from build123d import *
from build123d.topology import SkipClean

# Parameters (mm, degrees)
SKETCH2_W           = 31.75
SKETCH2_H           = 6.35
BOSS_EXTRUDE2_DEPTH = 31.75
SKETCH3_W           = 19.999999878
SKETCH3_H           = 40.64
CUT_EXTRUDE1_DEPTH  = 37.061067996
SKETCH4_R           = 1.63195
CUT_EXTRUDE2_DEPTH  = 37.061067996
SKETCH7_W           = 3.175
SKETCH7_H           = 1.905
SKETCH7_W_2         = 2.54
SKETCH7_H_2         = 3.175
CUT_EXTRUDE4_DEPTH  = 37.061067996
CHAMFER1_SIZE       = 1.27
CUT_EXTRUDE3_DEPTH  = 2.38125
BOSS_EXTRUDE5_DEPTH = 31.75
SKETCH12_W          = 19.999999878
SKETCH12_H          = 25.4
CUT_EXTRUDE5_DEPTH  = 81.946934778
BOSS_EXTRUDE6_DEPTH = 9.071430469
BOSS_EXTRUDE7_DEPTH = 9.071428449
BOSS_EXTRUDE8_DEPTH = 31.75
SKETCH16_W          = 19.999999878
SKETCH16_H          = 45.357142858
SKETCH18_W          = 19.999999878
SKETCH18_H          = 38.1


with BuildPart() as part:
    # Sketch2 → Boss-Extrude2 (new, symmetric)
    with BuildSketch(Plane.XY):
        Rectangle(SKETCH2_W, SKETCH2_H)
    extrude(amount=BOSS_EXTRUDE2_DEPTH, both=True)

    # Sketch3 → Cut-Extrude1 (cut, through all)
    with BuildSketch(Plane(origin=(0, 3.175, 0), x_dir=(1, 0, 0), z_dir=(0, 1, 0))):
        Rectangle(SKETCH3_W, SKETCH3_H)
    extrude(amount=-CUT_EXTRUDE1_DEPTH, mode=Mode.SUBTRACT)

    # Sketch4 → Cut-Extrude2 (cut, through all)
    with BuildSketch(Plane(origin=(0, 3.175, 0), x_dir=(1, 0, 0), z_dir=(0, 1, 0))):
        with Locations(Location((-5.08, 25.4, 0), (0, 0, 270))):
            Circle(SKETCH4_R)
        with Locations(Location((5.08, 25.4, 0), (0, 0, 270))):
            Circle(SKETCH4_R)
        with Locations(Location((-5.08, -25.4, 0), (0, 0, 270))):
            Circle(SKETCH4_R)
        with Locations(Location((5.08, -25.4, 0), (0, 0, 270))):
            Circle(SKETCH4_R)
    extrude(amount=-CUT_EXTRUDE2_DEPTH, mode=Mode.SUBTRACT)

    # Sketch7 → Cut-Extrude4 (cut, through all)
    with BuildSketch(Plane(origin=(0, 3.175, 0), x_dir=(1, 0, 0), z_dir=(0, 1, 0))):
        with Locations((-2.8575, 21.2725)):
            Rectangle(SKETCH7_W, SKETCH7_H)
        with Locations((2.8575, 21.2725)):
            Rectangle(SKETCH7_W, SKETCH7_H)
        with Locations((2.8575, -21.2725)):
            Rectangle(SKETCH7_W, SKETCH7_H)
        with Locations((-2.8575, -21.2725)):
            Rectangle(SKETCH7_W, SKETCH7_H)
        with Locations((0, 21.2725)):
            Rectangle(SKETCH7_W_2, SKETCH7_H)
        with Locations((0, 23.8125)):
            Rectangle(SKETCH7_W_2, SKETCH7_H_2)
        with Locations((0, -21.2725)):
            Rectangle(SKETCH7_W_2, SKETCH7_H)
        with Locations((0, -23.8125)):
            Rectangle(SKETCH7_W_2, SKETCH7_H_2)
    extrude(amount=-CUT_EXTRUDE4_DEPTH, mode=Mode.SUBTRACT)

    # Chamfer1
    chamfer1_edges = [part.edges().sort_by_distance(p)[0] for p in [
        (-4.445, 0, -22.225),
        (4.445, 0, -22.225),
        (4.445, 0, 22.225),
        (-4.445, 0, 22.225),
    ]]
    chamfer(chamfer1_edges, length=CHAMFER1_SIZE)

    # Sketch6 → Cut-Extrude3 (cut)
    with BuildSketch(Plane.XZ.offset(3.175)):
        Polygon((-1.905, 27.233087105), (-5.08, 29.066174209), (-8.255, 27.233087105), (-8.255, 23.566912895), (-5.08, 21.733825791), (-1.905, 23.566912895), align=None)
        Polygon((8.255, 27.233087105), (5.08, 29.066174209), (1.905, 27.233087105), (1.905, 23.566912895), (5.08, 21.733825791), (8.255, 23.566912895), align=None)
        Polygon((8.255, -23.566912895), (5.08, -21.733825791), (1.905, -23.566912895), (1.905, -27.233087105), (5.08, -29.066174209), (8.255, -27.233087105), align=None)
        Polygon((-1.905, -23.566912895), (-5.08, -21.733825791), (-8.255, -23.566912895), (-8.255, -27.233087105), (-5.08, -29.066174209), (-1.905, -27.233087105), align=None)
    extrude(amount=-CUT_EXTRUDE3_DEPTH, mode=Mode.SUBTRACT)

    # Sketch10 → Boss-Extrude5 (add, through all)
    with BuildSketch(Plane(origin=(15.875, 0, 0), x_dir=(0, 0, -1), z_dir=(1, 0, 0))):
        Polygon((25.4, -47.625), (19.05, -47.625), (19.05, -34.925), (-19.05, -34.925), (-19.05, -47.625), (-25.4, -47.625), (-31.75, -3.175), (-22.678571429, -3.175), (-19.05, -28.575), (19.05, -28.575), (22.678571429, -3.175), (31.75, -3.175), align=None)
    extrude(amount=-BOSS_EXTRUDE5_DEPTH)

    # Sketch12 → Cut-Extrude5 (cut, through all)
    with BuildSketch(Plane.XY.offset(31.75)):
        with Locations((0, -15.875)):
            Rectangle(SKETCH12_W, SKETCH12_H)
    extrude(amount=-CUT_EXTRUDE5_DEPTH, mode=Mode.SUBTRACT)

    # Sketch13 → Boss-Extrude6 (add, along a direction that is not the sketch's normal)
    with BuildSketch(Plane(origin=(0, -4.5085, -31.5595), x_dir=(-1, 0, 0), z_dir=(0, -0.14142135623730953, -0.9899494936611667))):
        Polygon((-9.999999939, -24.310836213), (0, -24.310836213), (-9.999999939, -14.310836274), align=None)
        Polygon((9.999999939, -14.310836274), (0, -24.310836213), (9.999999939, -24.310836213), align=None)
    extrude(amount=-BOSS_EXTRUDE6_DEPTH, dir=(0, 0, -1))

    # Sketch14 → Boss-Extrude7 (add, along a direction that is not the sketch's normal)
    with SkipClean():  # the faces are left unmerged after this step: merging them gives an invalid solid
        with BuildSketch(Plane(origin=(0, -4.5085, 31.5595), x_dir=(1, 0, 0), z_dir=(0, -0.14142135623730945, 0.9899494936611667))):
            Polygon((-9.999999939, -24.310836213), (0, -24.310836213), (-9.999999939, -14.310836274), align=None)
            Polygon((9.999999939, -14.310836274), (0, -24.310836213), (9.999999939, -24.310836213), align=None)
        extrude(amount=-BOSS_EXTRUDE7_DEPTH, dir=(0, 0, 1))

    # Sketch15 → Boss-Extrude8 (add)
    with BuildSketch(Plane(origin=(15.875, 0, 0), x_dir=(0, 0, -1), z_dir=(1, 0, 0))):
        Polygon((22.225, -6.35), (0, -28.575), (19.05, -28.575), align=None)
        Polygon((-19.05, -28.575), (0, -28.575), (-22.225, -6.35), align=None)
    extrude(amount=-BOSS_EXTRUDE8_DEPTH)

    # Sketch16 → Cut-Loft1 section 0
    with BuildSketch(Plane.XZ.offset(3.175)):
        Rectangle(SKETCH16_W, SKETCH16_H)
    # Sketch18 → Cut-Loft1 section 1
    with BuildSketch(Plane.XZ.offset(34.925)):
        Rectangle(SKETCH18_W, SKETCH18_H)
    loft(mode=Mode.SUBTRACT)


solid = part.part
Here's how the part is built. I have some questions about the finished solid (model axes, mm). A direction names the side the tool comes from. Give positions to 0.01 mm unless a question says otherwise; leave off trailing zeros. Order: outer loops, then holes, each group sorted by start corner. A loop starts at its lowest first (then second) coordinate and runs counter-clockwise, first axis right, second up. Notation, with made-up numbers: (53, 66.5) -> (112, 66.5) arc R34 ccw to (112, 100.5) -> close; hole circle Ø8 at (-20.75, 47). An arc over 180 degrees is marked (long way). One line per item, written item: value. Start each with the question number.
1. Imagine slicing it at B-B, the plane z = -11. List the corners of the cut face in (x, y) for me (3 decimals).
2. Imagine slicing it at C-C, the plane y = -11.5. List the corners of the cut face in (x, z) for me (3 decimals).
3. Imagine slicing it at D-D, the plane y = -32. List the corners of the cut face in (x, z) for me (3 decimals), plus the area to 3 significant figures.
4. For faces 5 (the face through (4.087, 1.218, -26.695)), 6 (the face through (-4.932, -23.693, 24.565)), 7 (the face through (3.47, -2.001, 22.663)), which set-ups out of +Z, -Z, +X, -X, +Y, -Y let a thin tool reach every point of the face, with its end or its side?
5. Imagine slicing it at A-A, the plane x = -11. List the corners of the cut face in (y, z) for me (3 decimals).
6. Will these pins go through, and if not, where does the flat tip stop? pin 1 Ø1.5 at (x, y) = (9.5, -20.5) entering from -Z; pin 2 Ø10 at (x, y) = (0, -44) entering from +Z; pin 3 Ø6.5 at (x, z) = (-12, -4) entering from -Y (3 decimals).
7. We'd pull the mould along Z, two halves only. Please class faces 1 (the face through (7, 0, -20.32)), 2 (the face through (0, 0, -31.75)), 3 (the face through (-3.51, -2, 22.64)), 4 (the face through (10.4, 3.175, 0.4)): released by +Z, released by -Z, zero draft, split by the parting line, or undercut.
8. I need wall thicknesses on probe 1 along Z at (x, y) = (-5, 2); probe 2 along X at (y, z) = (-33, -17.5) (3 decimals); probe 3 along X at (y, z) = (0, -25) (3 decimals). Which ranges of each line are inside material? Lowest first, please. Write a range as from..to.
Values follow:
1. outline: (-15.875, -34.925) -> (-10, -34.925) -> (-10, -17.575) -> (-15.875, -17.575) -> close; (-15.875, -3.175) -> (-10, -3.175) -> (-10, 3.175) -> (-15.875, 3.175) -> close; (10, -34.925) -> (15.875, -34.925) -> (15.875, -17.575) -> (10, -17.575) -> close; (10, -3.175) -> (15.875, -3.175) -> (15.875, 3.175) -> (10, 3.175) -> close
2. outline: (-15.875, -30.561) -> (-10, -30.561) -> (-10, -17.075) -> (-15.875, -17.075) -> close; (-15.875, 17.075) -> (-10, 17.075) -> (-10, 30.561) -> (-15.875, 30.561) -> close; (10, -30.561) -> (15.875, -30.561) -> (15.875, -17.075) -> (10, -17.075) -> close; (10, 17.075) -> (15.875, 17.075) -> (15.875, 30.561) -> (10, 30.561) -> close
3. outline: (-15.875, -27.632) -> (15.875, -27.632) -> (15.875, 27.632) -> (-15.875, 27.632) -> close; hole (-10, -19.384) -> (10, -19.384) -> (10, 19.384) -> (-10, 19.384) -> close
3. area: 979 mm2
4. face 5: +Y
4. face 6: +Z, -Z
4. face 7: none
5. outline: (-47.625, -25.4) -> (-3.175, -31.75) -> (3.175, -31.75) -> (3.175, 31.75) -> (-3.175, 31.75) -> (-47.625, 25.4) -> (-47.625, 19.05) -> (-34.925, 19.05) -> (-34.925, -19.05) -> (-47.625, -19.05) -> close; hole (-28.575, 0) -> (-6.35, -22.225) -> (-3.175, -22.679) -> (-3.175, 22.679) -> (-6.35, 22.225) -> close
6. pin 1: stops at z = -29.38
6. pin 2: stops at z = 26.63
6. pin 3: stops at y = -34.925
7. face 1: undercut
7. face 2: released by -Z
7. face 3: undercut
7. face 4: zero draft
8. probe 1: z = -31.75..-27.03, -23.77..-20.32, 20.32..23.77, 27.03..31.75
8. probe 2: x = -15.875..-10, 10..15.875
8. probe 3: x = -15.875..-6.662, -3.498..-1.27, 1.27..3.498, 6.662..15.875
